The model under review builds one solid part; all positions refer to its coordinate system, in mm. A direction names the side the tool comes from. Round coordinates to 2 decimals unless told otherwise and drop trailing zeros. Write each loop counter-clockwise with the first axis right and the second up, starting at its lowest first coordinate (ties: lowest second). Pieces come first, ordered by that corner, then holes. Notation, with made-up numbers: (19, 58) -> (61, 58) arc R14 ccw to (61, 64) -> close; hole circle Ø11 at (-36, 60). An arc over 180 degrees is marked (long way). Answer as a JSON object with one key per item and string values. Group by question number.
1) To check wall thickness, follow probe 1 along X at (y, z) = (13, 0); probe 2 along X at (y, z) = (-4, 4.25); probe 3 along Z at (x, y) = (-4.72, 13). State the ranges of each line that lie inside material, in increasing order. Write a range as [from, to].
2) Machinability: for faces 1 (the flat face through (0, -13, 7.5)), 2 (the flat face through (5, 7, -2)), 3 (the flat face through (8.67, -3.57, 3.61)), 4 (the cylindrical face through (-4.104, -16.873, -5.297)), which of the approach directions +Z, -Z, +X, -X, +Y, -Y give a long, thin tool a straight path to every point of the face, cutting with its end or side? Answer none if there is none.
3) We need section C-C, the plane y = -1. Write out the cut boundary in (x, z), then the cut area to 3 significant figures.
4) Mouldability with a two-part tool opening along X and no side actions: class faces 5 (the flat face through (-10.5, 0, 2)), 6 (the flat face through (2.33, -3.57, 3.61)), 7 (the flat face through (1, -4, 11.5)) as pulls with the +X half, pulls with the -X half, needs draft (parallel to the pull), parting line crosses it, or undercut.
5) We need section B-B, the plane z = -5.08. Write out the cut boundary in (x, y).
6) Insertion check: pin 1 Ø1.2 at (x, z) = (-2.5, 9.5) entering from +Y; pin 2 Ø1.4 at (x, y) = (4.5, -4.5) entering from +Z; pin 3 Ø1.4 at (x, z) = (-4.5, 1.5) entering from +Y. Each pin has a flat end and moves straight along its axis. Give the tip position at first contact, or say it passes through.
7) We need section A-A, the plane x = -0.5. Write out the cut boundary in (y, z).
8) We need section D-D, the plane z = 7. Write out the cut boundary in (x, y), then the cut area to 3 significant figures.
from build123d import *
from build123d.topology import SkipClean

# Parameters (mm, degrees)
SKETCH_1_W                    = 15
SKETCH_1_H                    = 30
SKETCH_1_W_2                  = 4
SKETCH_1_H_2                  = 13
EXTRUDE_1_DEPTH               = 10.5
SKETCH_3_R                    = 3.4
CUT_EXTRUDE_1_DEPTH           = 8
SKETCH_4_W                    = 8
SKETCH_4_H                    = 10
CUT_EXTRUDE_3_DEPTH           = 16
CUT_EXTRUDE_3_DRAFT           = -6
CUT_EXTRUDE_3_PROFILE_2_DEPTH = 16
CUT_EXTRUDE_3_PROFILE_2_DRAFT = -6
CUT_EXTRUDE_5_DEPTH           = 1
CUT_EXTRUDE_6_DEPTH           = 1
SKETCH_9_R                    = 1
EXTRUDE_2_DEPTH               = 4
FILLET_3_R                    = 0.2


with BuildPart() as part:
    # Эскиз1 → Бобышка-Вытянуть1 (new, symmetric)
    with BuildSketch(Plane(origin=(0, 0, 0), x_dir=(0, 0, -1), z_dir=(1, 0, 0))):
        Rectangle(SKETCH_1_W, SKETCH_1_H)
        with Locations((-9.5, -3.5)):
            Rectangle(SKETCH_1_W_2, SKETCH_1_H_2)
    extrude(amount=EXTRUDE_1_DEPTH, both=True)

    # Эскиз3 → Вырез-Вытянуть1 (cut)
    with BuildSketch(Plane(origin=(0, 15, 0), x_dir=(1, 0, 0), z_dir=(0, 1, 0))):
        with Locations(Location((-4.72, 0, 0), (0, 0, 270))):
            Circle(SKETCH_3_R)
        with Locations(Location((4.72, 0, 0), (0, 0, 270))):
            Circle(SKETCH_3_R)
    extrude(amount=-CUT_EXTRUDE_1_DEPTH, mode=Mode.SUBTRACT)


with BuildPart() as cut_extrude_3_tool:
    # Эскиз4 → Вырез-Вытянуть3 (with draft: the straight prism first)
    with BuildSketch(Plane.XY.offset(11.5)):
        with Locations((-5.5, -3.5)):
            Rectangle(SKETCH_4_W, SKETCH_4_H)
    extrude(amount=-CUT_EXTRUDE_3_DEPTH)
    # Вырез-Вытянуть3: the draft: its side faces are tilted about the plane it starts from
    cut_extrude_3_sides = [cut_extrude_3_tool.faces().sort_by_distance(p)[0] for p in [
        (-5.5, -8.5, 3.5),
        (-1.5, -3.5, 3.5),
        (-5.5, 1.5, 3.5),
        (-9.5, -3.5, 3.5),
    ]]
    draft(cut_extrude_3_sides, Plane.XY.offset(11.5), CUT_EXTRUDE_3_DRAFT)


with BuildPart() as part_1:
    add(part.part)

    # Вырез-Вытянуть3: cut by cut_extrude_3_tool
    add(cut_extrude_3_tool.part, mode=Mode.SUBTRACT)


with BuildPart() as cut_extrude_3_profile_2_tool:
    # Эскиз4 → Вырез-Вытянуть3 profile 2 (with draft: the straight prism first)
    with BuildSketch(Plane.XY.offset(11.5)):
        with Locations((5.5, -3.5)):
            Rectangle(SKETCH_4_W, SKETCH_4_H)
    extrude(amount=-CUT_EXTRUDE_3_PROFILE_2_DEPTH)
    # Вырез-Вытянуть3 profile 2: the draft: its side faces are tilted about the plane it starts from
    cut_extrude_3_profile_2_sides = [cut_extrude_3_profile_2_tool.faces().sort_by_distance(p)[0] for p in [
        (5.5, -8.5, 3.5),
        (9.5, -3.5, 3.5),
        (5.5, 1.5, 3.5),
        (1.5, -3.5, 3.5),
    ]]
    draft(cut_extrude_3_profile_2_sides, Plane.XY.offset(11.5), CUT_EXTRUDE_3_PROFILE_2_DRAFT)


with BuildPart() as part_2:
    add(part_1.part)

    # Вырез-Вытянуть3 profile 2: cut by cut_extrude_3_profile_2_tool
    add(cut_extrude_3_profile_2_tool.part, mode=Mode.SUBTRACT)

    # Эскиз7 → Вырез-Вытянуть5 (cut)
    with BuildSketch(Plane(origin=(0, 7, 0), x_dir=(1, 0, 0), z_dir=(0, 1, 0))):
        with BuildLine():
            ThreePointArc((-8.12, 1e-09), (-8.110745992, -0.250682298), (-8.083034344, -0.5))
            Line((-8.083034344, -0.5), (-1.356965656, -0.5))
            ThreePointArc((-1.356965656, -0.5), (-1.329254008, -0.250682299), (-1.32, 0))
            ThreePointArc((-1.32, 0), (-1.329254008, 0.250682299), (-1.356965656, 0.5))
            Line((-1.356965656, 0.5), (-8.083034344, 0.5))
            ThreePointArc((-8.083034344, 0.5), (-8.110745992, 0.250682299), (-8.12, 1e-09))
        make_face()
    extrude(amount=-CUT_EXTRUDE_5_DEPTH, mode=Mode.SUBTRACT)

    # Эскиз8 → Вырез-Вытянуть6 (cut)
    with SkipClean():  # the faces are left unmerged after this step: merging them gives an invalid solid
        with BuildSketch(Plane(origin=(0, 7, 0), x_dir=(1, 0, 0), z_dir=(0, 1, 0))):
            with BuildLine():
                Line((1.356965656, 0.5), (8.083034344, 0.5))
                ThreePointArc((8.083034344, 0.5), (8.12, 0), (8.083034344, -0.5))
                Line((8.083034344, -0.5), (1.356965656, -0.5))
                ThreePointArc((1.356965656, -0.5), (1.32, 0), (1.356965656, 0.5))
            make_face()
        extrude(amount=-CUT_EXTRUDE_6_DEPTH, mode=Mode.SUBTRACT)

    # Эскиз9 → Бобышка-Вытянуть2 (add)
    with SkipClean():  # the faces are left unmerged after this step: merging them gives an invalid solid
        with BuildSketch(Plane.XZ.offset(15)):
            with Locations(Location((-5.08, 5.08, 0), (0, 0, 90))):
                Circle(SKETCH_9_R)
            with Locations(Location((5.08, 5.08, 0), (0, 0, 90))):
                Circle(SKETCH_9_R)
            with Locations(Location((5.08, -5.08, 0), (0, 0, 90))):
                Circle(SKETCH_9_R)
            with Locations(Location((-5.08, -5.08, 0), (0, 0, 90))):
                Circle(SKETCH_9_R)
        extrude(amount=EXTRUDE_2_DEPTH)

    # Скругление3
    fillet_3_edges = [part_2.edges().sort_by_distance(p)[0] for p in [
        (-5.08, -19, -6.08),
        (-5.08, -19, 4.08),
        (5.08, -19, 4.08),
        (5.08, -19, -6.08),
    ]]
    fillet(fillet_3_edges, radius=FILLET_3_R)


solid = part_2.part
Here are the results:
{
 "1": {"probe 1": "x = [-10.5, -8.12], [-1.32, 1.32], [8.12, 10.5]", "probe 2": "x = [-10.5, -8.74], [-2.26, 2.26], [8.74, 10.5]", "probe 3": "z = [-7.5, -3.4], [3.4, 7.5]"},
 "2": {"face 1": "+Z, +X, -X, -Y", "face 2": "+Y", "face 3": "+Z", "face 4": "-Y"},
 "3": {"outline": "(-10.5, -7.5) -> (10.5, -7.5) -> (10.5, 11.5) -> (9.5, 11.5) -> (7.82, -4.5) -> (3.18, -4.5) -> (1.5, 11.5) -> (-1.5, 11.5) -> (-3.18, -4.5) -> (-7.82, -4.5) -> (-9.5, 11.5) -> (-10.5, 11.5) -> close", "area": "197 mm^2"},
 "4": {"face 5": "pulls with the -X half", "face 6": "undercut", "face 7": "needs draft"},
 "5": {"outline": "(-10.5, -15) -> (-6.08, -15) -> (-6.08, -18.8) arc R0.2 ccw to (-5.88, -19) -> (-4.28, -19) arc R0.2 ccw to (-4.08, -18.8) -> (-4.08, -15) -> (4.08, -15) -> (4.08, -18.8) arc R0.2 ccw to (4.28, -19) -> (5.88, -19) arc R0.2 ccw to (6.08, -18.8) -> (6.08, -15) -> (10.5, -15) -> (10.5, 15) -> (-10.5, 15) -> close"},
 "6": {"pin 1": "stops at y = 3", "pin 2": "stops at z = -4.5", "pin 3": "stops at y = 7"},
 "7": {"outline": "(-15, -7.5) -> (15, -7.5) -> (15, 7.5) -> (3, 7.5) -> (3, 11.5) -> (-10, 11.5) -> (-10, 7.5) -> (-15, 7.5) -> close"},
 "8": {"outline": "(-10.5, -15) -> (10.5, -15) -> (10.5, 15) -> (-10.5, 15) -> close; hole (-9.03, -8.03) -> (-1.97, -8.03) -> (-1.97, 1.03) -> (-9.03, 1.03) -> close; hole (1.97, -8.03) -> (9.03, -8.03) -> (9.03, 1.03) -> (1.97, 1.03) -> close", "area": "502 mm^2"}
}
